Geometry check sheet. Reference: drawing and pictorial views, mm from the part's lowest x, y, z. A direction names the side the tool comes from. Round coordinates to 2 decimals unless told otherwise and drop trailing zeros. Order: outer loops, then holes, each group sorted by start corner. A loop starts at its lowest first (then second) coordinate and runs counter-clockwise, first axis right, second up.
Q1. Depth check by flat-ended pin: P1, Ø1, axis at y = 2, z = 3.5, coming from the -X side; P2, Ø1, axis at x = 2, z = 2, coming from the -Y side. Enter the tip coordinate at first touch or a pass-through.
Q2. Scan lines: probe 1 along Y at (x, z) = (14.75, 2.3); probe 2 along Z at (x, y) = (12.5, 16); probe 3 along X at (y, z) = (16.25, 1.95). Record each from-to range of solid material in increasing order.
Q3. Set-up check for the marked faces 1 and 2: record each of +Z, -Z, +X, -X, +Y, -Y from which the full face is reachable in a straight line by a thin tool's end or side.
Q4. Cross-section at A-A on y = 9. Record the cut outline in (x, z), then the cut area to 3 significant figures.
Q5. Cross-section at C-C on z = 1.5. Record the cut outline in (x, y), then the cut area to 3 significant figures.
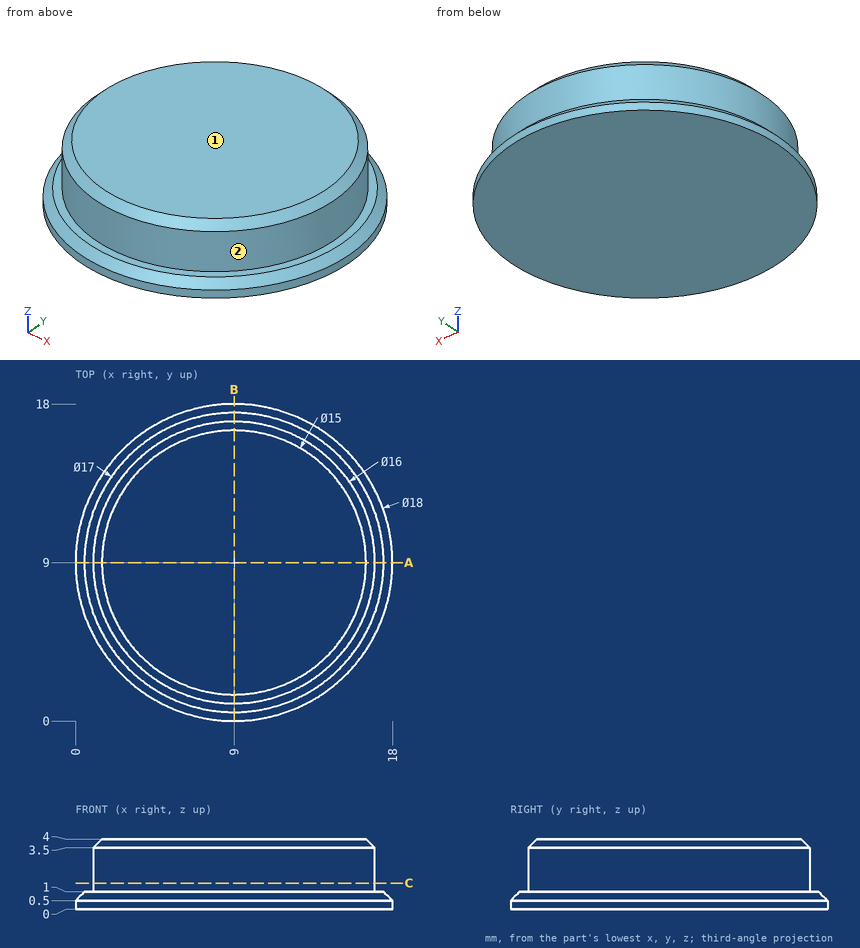
Results found:
1. P1: stops at x = 4.34
1. P2: stops at y = 4.34
2. probe 1: y = 3.44 to 14.56
2. probe 2: z = 0 to 3.67
2. probe 3: x = 5.62 to 12.38
3. face 1: +Z, +X, -X, +Y, -Y
3. face 2: +Z
4. outline: (0, 0) - (18, 0) - (18, 0.5) - (17.5, 1) - (17, 1) - (17, 3.5) - (16.5, 4) - (1.5, 4) - (1, 3.5) - (1, 1) - (0.5, 1) - (0, 0.5) - close
4. area: 65.5 mm2
5. outline: circle Ø16 at (9, 9)
5. area: 201 mm2
